Check sheet for the modelled part. Datum: model origin and axes. Units: mm. Face numbers are marked on the shaded views. A direction names the side the tool comes from. Round coordinates to 2 decimals unless told otherwise and drop trailing zeros. Order: outer loops, then holes, each group sorted by start corner. A loop starts at its lowest first (then second) coordinate and runs counter-clockwise, first axis right, second up. Notation, with made-up numbers: (-32.75, 27.5) -> (-16.75, 27.5) arc R22 cw to (-16.75, 48.5) -> close; hole circle Ø7 at (-36, 81.25). An arc over 180 degrees is marked (long way). Answer in a Markdown table with one row per item. Add a question column.
1. Sectioned sample at A-A, the plane z = -38.5. Count the separate pieces of the cut face and the enclosed holes in it, then the cut area to 3 significant figures.
2. Draft check along X on the marked faces 3, 4 and 5. Enter one of: +X half, -X half, draft (parallel to the pull), parting line (faces both ways), or undercut.
3. Depth check by flat-ended pin: P1, Ø20, axis at x = -260, y = -17.5, coming from the -Z side; P2, Ø12, axis at x = -276.5, z = -30.5, coming from the -Y side. Enter the tip coordinate at first touch or a pass-through.
4. Material ranges on L1, parallel to Z at x = 221, y = -48, recorded low to high. Write a range as from..to.
5. Sectioned sample at B-B, the plane x = 169. Record the boundary of the cut face in (y, z), then the cut area to 3 significant figures.
6. Access from +Z, -Z, +X, -X, +Y, -Y to the whole of each face (thin tool, end or side, straight path). Record for the marked faces 1 and 2.
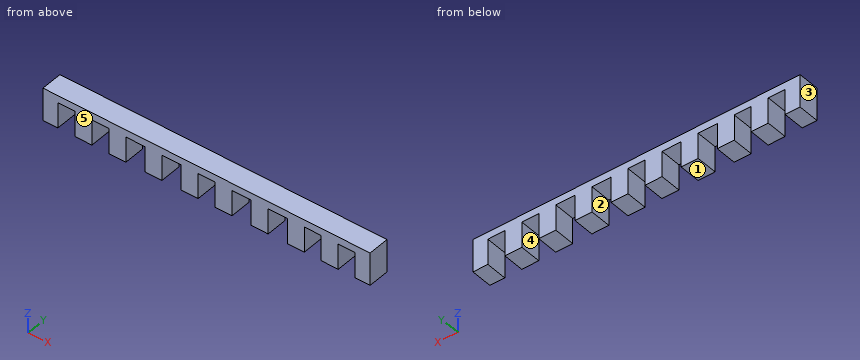
```python
from build123d import *

# Parameters (mm, degrees)
F0_W     = 780
F0_H     = 80
F1_DEPTH = 50
F2_W     = 40
F2_H     = 60
F2_W_2   = 45
F3_DEPTH = 50
F4_W     = 780
F4_H     = 3
F5_DEPTH = 50
F6_W     = 5
F6_H     = 77
F7_DEPTH = 50
F8_W     = 5
F8_H     = 77
F9_DEPTH = 50


with BuildPart() as f1:
    # F0 (on Front) → F1 (new body)
    with BuildSketch(Plane.XZ):
        with Locations((-14.780855, -40)):
            Rectangle(F0_W, F0_H)
    extrude(amount=F1_DEPTH)

    # F2 (on face) → F3 (cut)
    with BuildSketch(Plane.XZ.offset(50)):
        with Locations((-344.780855, -50)):
            Rectangle(F2_W, F2_H)
        with Locations((-264.780855, -50)):
            Rectangle(F2_W, F2_H)
        with Locations((-182.280855, -50)):
            Rectangle(F2_W_2, F2_H)
        with Locations((-97.280855, -50)):
            Rectangle(F2_W_2, F2_H)
        with Locations((-14.780855, -50)):
            Rectangle(F2_W, F2_H)
        with Locations((67.719145, -50)):
            Rectangle(F2_W_2, F2_H)
        with Locations((152.719145, -50)):
            Rectangle(F2_W_2, F2_H)
        with Locations((235.219145, -50)):
            Rectangle(F2_W, F2_H)
        with Locations((315.219145, -50)):
            Rectangle(F2_W, F2_H)
    extrude(amount=-F3_DEPTH, mode=Mode.SUBTRACT)

    # F4 (on face) → F5 (cut, through all)
    with BuildSketch(Plane.XZ.offset(50)):
        with Locations((-14.780855, -1.5)):
            Rectangle(F4_W, F4_H)
    extrude(amount=-F5_DEPTH, mode=Mode.SUBTRACT)

    # F6 (on face) → F7 (cut, through all)
    with BuildSketch(Plane.XZ.offset(50)):
        with Locations((-402.280855, -41.5)):
            Rectangle(F6_W, F6_H)
    extrude(amount=-F7_DEPTH, mode=Mode.SUBTRACT)

    # F8 (on face) → F9 (cut, through all)
    with BuildSketch(Plane.XZ.offset(50)):
        with Locations((372.719145, -41.5)):
            Rectangle(F8_W, F8_H)
    extrude(amount=-F9_DEPTH, mode=Mode.SUBTRACT)


solid = f1.part
```
Answer key:
| question | item | result |
|---|---|---|
| 1 | separate pieces | 10 |
| 1 | enclosed holes | 0 |
| 1 | area | 19,500 mm² |
| 2 | face 3 | -X half |
| 2 | face 4 | undercut |
| 2 | face 5 | draft |
| 3 | P1 | stops at z = -20 |
| 3 | P2 | passes through |
| 4 | L1 | z = -20..-3 |
| 5 | outline | (-50, -20) -> (0, -20) -> (0, -3) -> (-50, -3) -> close |
| 5 | area | 850 mm² |
| 6 | face 1 | -Z, +X, -X, +Y, -Y |
| 6 | face 2 | -Z, +Y, -Y |
